Autodesk Inventor part; units mm, degrees
ref_plane "YZ Plane" through (0, 0, 0) normal (1, 0, 0) x (0, 1, 0)
ref_plane "XZ Plane" through (0, 0, 0) normal (0, 1, 0) x (-1, 0, 0)
ref_plane "XY Plane" through (0, 0, 0) normal (0, 0, 1) x (1, 0, 0)
sketch "Esquisse1" plane through (0, 0, 0) normal (0, 0, 1) x (1, 0, 0)
  line L0 (-21, -21) -> (21, -21)
  line L1 (21, -21) -> (21, 21)
  line L2 (21, 21) -> (-21, 21)
  line L3 (-21, 21) -> (-21, -21)
  line L4 (-21, -21) -> (21, 21) construction
  line L5 (21, -21) -> (-21, 21) construction
  point P0 (0, 0)
  dimension "d0" = 42
  dimension "d1" = 42
extrude "Extrusion1" add sketch "Esquisse1" along normal mid plane 20.5
sketch "Esquisse2" plane through (0, 0, 10.25) normal (0, 0, 1) x (1, 0, 0)
  point P0 (0, 0)
  point P1 (0, 0)
hole "Perçage1" at (0, 0, 10.25) direction (0, 0, -1) diameter 36.5 end through all
sketch "Esquisse3" plane through (0, 0, 10.25) normal (0, 0, 1) x (1, 0, 0)
  point P0 (0, 0)
  point P1 (-15.625, 15.625)
  point P2 (-15.625, -15.625)
  point P3 (15.625, -15.625)
  point P4 (15.625, 15.625)
  dimension "d11" = 31.25
  dimension "d12" = 31.25
  dimension "d13" = 15.625
  dimension "d14" = 15.625
hole "Perçage2" at (-15.625, 15.625, 10.25) at (-15.625, -15.625, 10.25) at (15.625, -15.625, 10.25) at (15.625, 15.625, 10.25) direction (0, 0, -1) diameter 3.5 end through all
chamfer "Chanfrein1" distance 5 angle 45 4 edges at (21, 21, 0) (-21, 21, 0) (21, -21, 0) (-21, -21, 0)
chamfer "Chanfrein2" distance 0.5 angle 45 17 edges at (-21, 0, 10.25) (-18.5, -18.5, 10.25) (0, -21, 10.25) (18.5, -18.5, 10.25) (21, 0, 10.25) (18.5, 18.5, 10.25) (0, 21, 10.25) (0, 18.25, 10.25) (-18.5, 18.5, -10.25) (0, 21, -10.25) (0, 18.25, -10.25) (-21, 0, -10.25) (0, -21, -10.25) (-18.5, -18.5, -10.25) (18.5, -18.5, -10.25) (21, 0, -10.25) (18.5, 18.5, -10.25)
properties part number "Cache reducteur" material "----------"
Input: part model. Units: mm. Frame: model coordinates. Give positions to 0.01 mm unless a question says otherwise; leave off trailing zeros. Order: outer loops, then holes, each group sorted by start corner. A loop starts at its lowest first (then second) coordinate and runs counter-clockwise, first axis right, second up.
1. Line query: probe 1 along X at (y, z) = (0, 2.25); probe 2 along X at (y, z) = (-16, -9). Output: solid intervals per line, ascending.
Computed:
probe 1: x = -21 to -18.25, 18.25 to 21
probe 2: x = -21 to -17.33, -13.92 to -8.78, 8.78 to 13.92, 17.33 to 21
2. Cut plane C-C (z = 5.25). Return loops of the section in (x, y) (3 decimals), and give its area (3 significant figures).
Computed:
outline: (-21, -16) - (-16, -21) - (16, -21) - (21, -16) - (21, 16) - (16, 21) - (-16, 21) - (-21, 16) - close; hole circle Ø36.5 at (0, 0); hole circle Ø3.5 at (-15.625, -15.625); hole circle Ø3.5 at (-15.625, 15.625); hole circle Ø3.5 at (15.625, -15.625); hole circle Ø3.5 at (15.625, 15.625)
area: 629 mm2
3. Draft query along Y for faces 1 (the face through (-9, -17, -10.25)), 2 (the face through (18.36, 18.29, -10)), 3 (the face through (-17.1, 14.68, -0.14)), 4 (the face through (18.29, -18.36, -10)). Return one class per face: released by +Y, released by -Y, zero draft, split by the parting line, or undercut.
Computed:
face 1: zero draft
face 2: released by +Y
face 3: undercut
face 4: released by -Y
4. Cut plane D-D (x = -15). State how many separate pieces and enclosed holes the cut face has, and give its area (3 significant figures).
Computed:
separate pieces: 4
enclosed holes: 0
area: 299 mm2
5. Cut plane A-A (y = 0). Return loops of the section in (x, z), and give its area (3 significant figures).
Computed:
outline: (-21, -9.75) - (-20.5, -10.25) - (-18.75, -10.25) - (-18.25, -9.75) - (-18.25, 9.75) - (-18.75, 10.25) - (-20.5, 10.25) - (-21, 9.75) - close; (18.25, -9.75) - (18.75, -10.25) - (20.5, -10.25) - (21, -9.75) - (21, 9.75) - (20.5, 10.25) - (18.75, 10.25) - (18.25, 9.75) - close
area: 112 mm2
